For this review, use the dimensioned drawing (mm, ordinates from the lowest corner) and the shaded views. A direction names the side the tool comes from. Coordinates: 2 decimals unless noted, no trailing zeros. Write each loop counter-clockwise with the first axis right and the second up, starting at its lowest first coordinate (ties: lowest second). Pieces come first, ordered by that corner, then holes. Notation, with made-up numbers: (39, 79.25) -> (78, 79.25) arc R21 ccw to (78, 109.25) -> close; hole circle Ø10 at (77, 64.5). An arc over 180 degrees is marked (long way). Put each result on its own line as item: value. Start each with the question number.
Item 1: To check wall thickness, follow L1, parallel to X at y = 7, z = 53; L2, parallel to X at y = 23.5, z = 19.5; L3, parallel to X at y = 38, z = 57.2. State the ranges of each line that lie inside material, in increasing order.
Item 2: Consider section A-A on x = 14.5. Give the boundary of the cut face in (y, z).
Item 3: For the marked faces 4, 5 and 6, list the 3-axis set-ups (+Z, -Z, +X, -X, +Y, -Y) from which the entire face can be reached by the end or side of a thin tool; tool diameter is ignored.
Item 4: Consider section C-C on z = 7.5. Give the boundary of the cut face in (x, y).
Item 5: Insertion check: P1, Ø2, axis at x = 58, z = 47.5, coming from the +Y side; P2, Ø3.5, axis at y = 5.5, z = 55.5, coming from the +X side; P3, Ø6, axis at x = 3, z = 40.5, coming from the -Y side; P4, Ø3, axis at y = 7, z = 21.5, coming from the +X side. Each pin has a flat end and moves straight along its axis. Give the tip position at first contact, or say it passes through.
Item 6: Consider section B-B on y = 7. Give the boundary of the cut face in (x, z).
Item 7: The part is to be moulded in two halves that separate along Y. For the marked faces 1, 2 and 3, say which applies: +Y half, -Y half, draft (parallel to the pull), parting line (faces both ways), or undercut.
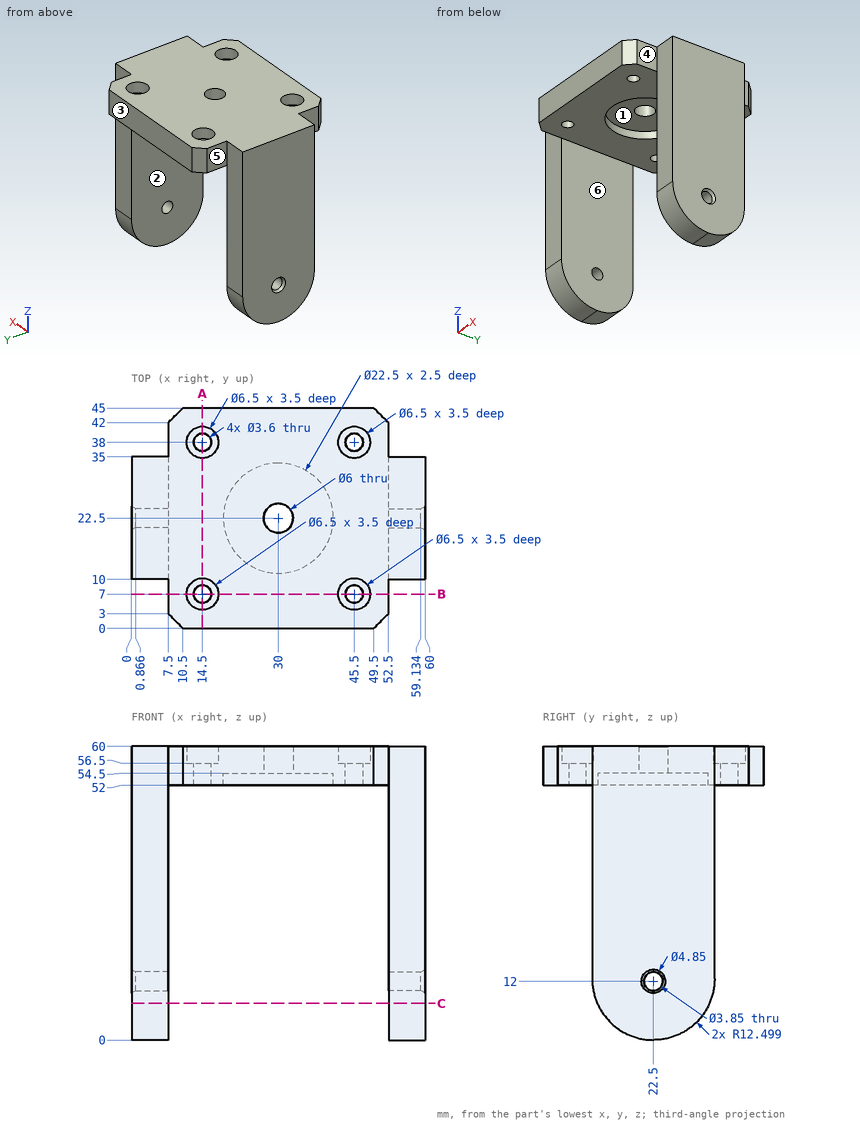
Return value:
1. L1: 7.5 to 12.7, 16.3 to 43.7, 47.3 to 52.5
1. L2: 0 to 7.5, 52.5 to 60
1. L3: 7.5 to 11.25, 17.75 to 42.25, 48.75 to 52.5
2. outline: (0, 52) -> (5.2, 52) -> (5.2, 56.5) -> (3.75, 56.5) -> (3.75, 60) -> (0, 60) -> close; (8.8, 52) -> (36.2, 52) -> (36.2, 56.5) -> (34.75, 56.5) -> (34.75, 60) -> (10.25, 60) -> (10.25, 56.5) -> (8.8, 56.5) -> close; (39.8, 52) -> (45, 52) -> (45, 60) -> (41.25, 60) -> (41.25, 56.5) -> (39.8, 56.5) -> close
3. face 4: +Z, -Z, +X, -Y
3. face 5: +Z, -Z, -X, +Y
3. face 6: -Z, +Y, -Y
4. outline: (0, 11.04) -> (7.5, 11.04) -> (7.5, 33.96) -> (0, 33.96) -> close; (52.5, 11.04) -> (60, 11.04) -> (60, 33.96) -> (52.5, 33.96) -> close
5. P1: y = 35
5. P2: x = 52.5
5. P3: y = 10
5. P4: through
6. outline: (7.5, 52) -> (12.7, 52) -> (12.7, 56.5) -> (11.25, 56.5) -> (11.25, 60) -> (7.5, 60) -> close; (16.3, 52) -> (43.7, 52) -> (43.7, 56.5) -> (42.25, 56.5) -> (42.25, 60) -> (17.75, 60) -> (17.75, 56.5) -> (16.3, 56.5) -> close; (47.3, 52) -> (52.5, 52) -> (52.5, 60) -> (48.75, 60) -> (48.75, 56.5) -> (47.3, 56.5) -> close
7. face 1: undercut
7. face 2: draft
7. face 3: +Y half
